```python
from build123d import *

# Parameters (mm, degrees)
SKETCH_W        = 62
SKETCH_H        = 39
PAD_DEPTH       = 2
SKETCH001_W     = 22
SKETCH001_H     = 13
POCKET_DEPTH    = 2.001
SKETCH002_R     = 2.5
POCKET001_DEPTH = 5
SKETCH003_R     = 2.5
POCKET002_DEPTH = 5


with BuildPart() as part:
    # Sketch → Pad (new body)
    with BuildSketch(Plane.XY):
        with Locations((31, 19.5)):
            Rectangle(SKETCH_W, SKETCH_H)
    extrude(amount=PAD_DEPTH)

    # Sketch001 (on Face6 of Pad) → Pocket (cut, through all)
    with BuildSketch(Plane.XY.offset(2)):
        with Locations((31, 21.5)):
            Rectangle(SKETCH001_W, SKETCH001_H)
    extrude(amount=-POCKET_DEPTH, mode=Mode.SUBTRACT)

    # Sketch002 (on Face5 of Pocket) → Pocket001 (cut)
    with BuildSketch(Plane.XY.offset(2)):
        with Locations((50, 32)):
            Circle(SKETCH002_R)
    extrude(amount=-POCKET001_DEPTH, mode=Mode.SUBTRACT)

    # Sketch003 (on Face5 of Pocket001) → Pocket002 (cut)
    with BuildSketch(Plane.XY.offset(2)):
        with Locations((50, 14)):
            Circle(SKETCH003_R)
    extrude(amount=-POCKET002_DEPTH, mode=Mode.SUBTRACT)


solid = part.part
```
The model under review builds one solid part; all positions refer to its coordinate system, in mm. A direction names the side the tool comes from. Round coordinates to 2 decimals unless told otherwise and drop trailing zeros. Loops run counter-clockwise (first coordinate to the right, second up) from the corner with the lowest first, then second, coordinate; pieces in that order, holes last.
Item 1: Take a section at A-A (y = 22.5). Write out the cut boundary in (x, z), then the cut area to 3 significant figures.
Determined:
outline: (0, 0) - (20, 0) - (20, 2) - (0, 2) - close; (42, 0) - (62, 0) - (62, 2) - (42, 2) - close
area: 80.0 mm2
Item 2: Take a section at B-B (x = 38). Write out the cut boundary in (y, z), then the cut area to 3 significant figures.
Determined:
outline: (0, 0) - (15, 0) - (15, 2) - (0, 2) - close; (28, 0) - (39, 0) - (39, 2) - (28, 2) - close
area: 52.0 mm2
Item 3: For line 1 (Y direction, x = 50, z = 0.75); line 2 (X direction, y = 26, z = 1.5); line 3 (X direction, y = 15.5, z = 0.8), list the stretches that pass through material, from the lowest coordinate up.
Determined:
line 1: y = 0 to 11.5, 16.5 to 29.5, 34.5 to 39
line 2: x = 0 to 20, 42 to 62
line 3: x = 0 to 20, 42 to 48, 52 to 62
Item 4: Mouldability with a two-part tool opening along X and no side actions: class faces 3 (the face through (31, 11, 0)), 4 (the face through (42, 21, 1)), 5 (the face through (62, 19, 1)) as released by +X, released by -X, zero draft, split by the parting line, or undercut.
Determined:
face 3: zero draft
face 4: undercut
face 5: released by +X
Item 5: Take a section at D-D (x = 50). Write out the cut boundary in (y, z), then the cut area to 3 significant figures.
Determined:
outline: (0, 0) - (11.5, 0) - (11.5, 2) - (0, 2) - close; (16.5, 0) - (29.5, 0) - (29.5, 2) - (16.5, 2) - close; (34.5, 0) - (39, 0) - (39, 2) - (34.5, 2) - close
area: 58.0 mm2
Item 6: For faces 1 (the face through (31, 15, 1)), 2 (the face through (0, 19, 1)), list the 3-axis set-ups (+Z, -Z, +X, -X, +Y, -Y) from which the entire face can be reached by the end or side of a thin tool; tool diameter is ignored.
Determined:
face 1: +Z, -Z
face 2: +Z, -Z, -X, +Y, -Y
Item 7: Take a section at C-C (z = 1.3). Write out the cut boundary in (x, y), then the cut area to 3 significant figures.
Determined:
outline: (0, 0) - (62, 0) - (62, 39) - (0, 39) - close; hole (20, 15) - (42, 15) - (42, 28) - (20, 28) - close; hole circle Ø5 at (50, 14); hole circle Ø5 at (50, 32)
area: 2,090 mm2
